from build123d import *

# Parameters (mm, degrees)
ESQUISSE1_W             = 30
ESQUISSE1_H             = 11
BOSS_EXTRU_1_DEPTH      = 16.2
BOSS_EXTRU_2_DEPTH      = 9.1
ESQUISSE3_W             = 33.4
ESQUISSE3_H             = 14
BOSS_EXTRU_3_DEPTH      = 2
CONG_1_R                = 3.5
ENL_V_MAT_EXTRU_1_DEPTH = 0.5


with BuildPart() as part:
    # Esquisse1 → Boss.-Extru.1 (new body)
    with BuildSketch(Plane.XY):
        Rectangle(ESQUISSE1_W, ESQUISSE1_H)
    extrude(amount=BOSS_EXTRU_1_DEPTH)

    # Esquisse2 → Boss.-Extru.2 (add)
    with BuildSketch(Plane(origin=(0, 0, 0), x_dir=(-1, 0, 0), z_dir=(0, 0, -1))):
        Polygon((-9.520156546, -2.694554874), (-13.5, 2.189177928), (-12.879843454, 2.694554874), (-8.9, -2.189177928), align=None)
        Polygon((-0.320156546, -2.694554874), (-4.3, 2.189177928), (-3.679843454, 2.694554874), (0.3, -2.189177928), align=None)
    extrude(amount=BOSS_EXTRU_2_DEPTH)

    # Esquisse3 → Boss.-Extru.3 (add)
    with BuildSketch(Plane.XY.offset(16.2)):
        Rectangle(ESQUISSE3_W, ESQUISSE3_H)
    extrude(amount=BOSS_EXTRU_3_DEPTH)

    # Congé1
    cong_1_edges = [part.edges().sort_by_distance(p)[0] for p in [
        (16.7, -7, 17.2),
        (16.7, 7, 17.2),
        (-16.7, 7, 17.2),
        (-16.7, -7, 17.2),
    ]]
    fillet(cong_1_edges, radius=CONG_1_R)

    # Esquisse5 → Enlèv. mat.-Extru.1 (cut)
    # profile 1 of 2: a face of its own
    with BuildSketch(Plane.XY.offset(18.2)):
        with BuildLine():
            add(Edge.make_bspline(
                [(-8.672344116, -3.115384615), (-8.816594542, -3.11454114), (-9.096803073, -3.112902677), (-9.505106438, -3.094675309), (-9.888147182, -3.064395858), (-10.245943635, -3.022899755), (-10.578588179, -2.972402097), (-10.885191819, -2.904990826), (-11.167173735, -2.828329399), (-11.425453052, -2.739480033), (-11.663510816, -2.639226475), (-11.885744181, -2.530107135), (-12.0918336, -2.40780713), (-12.285008724, -2.279261226), (-12.462319222, -2.139465144), (-12.62580805, -1.99141638), (-12.774096473, -1.832153938), (-12.907286041, -1.663222517), (-13.024073857, -1.485767046), (-13.127578093, -1.304636715), (-13.212833981, -1.116595132), (-13.282575645, -0.924117757), (-13.339507374, -0.72679892), (-13.378613639, -0.524688996), (-13.403175484, -0.317319479), (-13.405526699, -0.177353753), (-13.406719116, -0.106370192)],
                knots=[0, 0, 0, 0, 1.646148282, 3.197666765, 4.66315463, 6.030252048, 7.307778049, 8.501004361, 9.610818041, 10.641065266, 11.615491391, 12.557119604, 13.464013759, 14.348536654, 15.203310953, 16.038349431, 16.863300206, 17.683791446, 18.490318933, 19.285717724, 20.06220424, 20.843281102, 21.620494212, 22.403315558, 23.190242141, 24, 24, 24, 24], degree=3))
            add(Edge.make_bspline(
                [(-13.406719116, -0.106370192), (-13.405725902, -0.034758535), (-13.403749756, 0.107723458), (-13.375934308, 0.317616697), (-13.340032104, 0.523853953), (-13.28245088, 0.7233062), (-13.213547479, 0.919744698), (-13.122630536, 1.108284414), (-13.0237513, 1.295581798), (-12.90312695, 1.47312818), (-12.769817193, 1.646228322), (-12.618476538, 1.808491632), (-12.453293353, 1.964065993), (-12.270583572, 2.107075425), (-12.073148677, 2.243649111), (-11.859333594, 2.368602577), (-11.629612167, 2.484534626), (-11.385049352, 2.593624475), (-11.119112495, 2.689020666), (-10.833460316, 2.773835506), (-10.525506096, 2.843355619), (-10.196965336, 2.90084753), (-9.846210449, 2.945472196), (-9.473952104, 2.977949275), (-9.079957413, 2.995110587), (-8.810580002, 2.99834183), (-8.672344116, 3)],
                knots=[0, 0, 0, 0, 0.810910589, 1.61342667, 2.396193133, 3.181089899, 3.963115317, 4.752255436, 5.550715454, 6.36105385, 7.181178335, 8.024612154, 8.872680183, 9.750181803, 10.651284446, 11.591556747, 12.554036451, 13.566402641, 14.62422919, 15.753422176, 16.94128843, 18.199818041, 19.531985927, 20.947085226, 22.433341622, 24, 24, 24, 24], degree=3))
            add(Edge.make_bspline(
                [(-8.672344116, 3), (-8.534712415, 2.998305349), (-8.265942373, 2.994995999), (-7.873701987, 2.978317337), (-7.503450196, 2.944678932), (-7.154792256, 2.903215364), (-6.827566515, 2.845080871), (-6.521986194, 2.775033615), (-6.2369694, 2.695225184), (-5.974558239, 2.598364918), (-5.730419815, 2.491814224), (-5.502387515, 2.376006578), (-5.288628898, 2.251758245), (-5.090673237, 2.117232847), (-4.908696823, 1.971871056), (-4.74294709, 1.816405738), (-4.590643844, 1.652725679), (-4.455865409, 1.478616394), (-4.334322685, 1.299416276), (-4.231855178, 1.112099864), (-4.143073095, 0.921461088), (-4.070485552, 0.725596603), (-4.014193065, 0.524808811), (-3.975495046, 0.318430198), (-3.948293311, 0.107693838), (-3.9462218, -0.034768443), (-3.945180655, -0.106370192)],
                knots=[0, 0, 0, 0, 1.561645053, 3.049612875, 4.452756685, 5.778837748, 7.032101753, 8.221335837, 9.334924186, 10.387562255, 11.392109817, 12.355697819, 13.287721948, 14.19548756, 15.068665045, 15.927346723, 16.771751757, 17.602390507, 18.423119567, 19.225778204, 20.022010933, 20.807278863, 21.593079439, 22.384715467, 23.188155646, 24, 24, 24, 24], degree=3))
            add(Edge.make_bspline(
                [(-3.945180655, -0.106370192), (-3.946379855, -0.1773522), (-3.948744442, -0.317314863), (-3.973208323, -0.524706815), (-4.012539618, -0.726004524), (-4.067610881, -0.922201329), (-4.13502048, -1.114303766), (-4.22284416, -1.299694332), (-4.323989205, -1.480433653), (-4.439176304, -1.65604218), (-4.571150652, -1.823209934), (-4.717099564, -1.982916346), (-4.880765666, -2.131001619), (-5.059572209, -2.269585542), (-5.253034743, -2.399490408), (-5.461283099, -2.520733579), (-5.684672864, -2.632141235), (-5.924612019, -2.734107607), (-6.184724486, -2.824512173), (-6.467425199, -2.904059364), (-6.775585556, -2.967591262), (-7.107640965, -3.021444367), (-7.464266137, -3.064597565), (-7.845590095, -3.094662735), (-8.250888737, -3.11288884), (-8.529295376, -3.114537509), (-8.672344116, -3.115384615)],
                knots=[0, 0, 0, 0, 0.810927267, 1.598990287, 2.382942141, 3.152806972, 3.926217614, 4.706701772, 5.493896336, 6.292070767, 7.104102563, 7.925577746, 8.761822141, 9.623241997, 10.509042271, 11.423174113, 12.375371989, 13.360203808, 14.400680605, 15.520553799, 16.714061498, 17.994519714, 19.364400916, 20.818312473, 22.365209998, 24, 24, 24, 24], degree=3))
        make_face()
        with BuildLine():
            add(Edge.make_bspline(
                [(-8.675949886, -2.307692308), (-8.555739426, -2.307378423), (-8.32243453, -2.306769235), (-7.984001554, -2.291315187), (-7.667814755, -2.269804728), (-7.373997537, -2.242743333), (-7.103576783, -2.202215046), (-6.855428255, -2.156233227), (-6.630011273, -2.10108084), (-6.425355958, -2.035503901), (-6.238564308, -1.960805385), (-6.064657667, -1.879390931), (-5.901574914, -1.791153635), (-5.749711712, -1.694284826), (-5.610924423, -1.58686934), (-5.481695105, -1.47388697), (-5.366518241, -1.350247925), (-5.228358565, -1.179245905), (-5.085597394, -0.953479952), (-4.961278178, -0.669028437), (-4.883152037, -0.376737863), (-4.873216642, -0.17834897), (-4.868257578, -0.079326923)],
                knots=[0, 0, 0, 0, 1.459098681, 2.831824031, 4.11146945, 5.306290378, 6.412266529, 7.42953815, 8.369053297, 9.227277979, 10.03601793, 10.809473603, 11.557037441, 12.285528272, 12.993193355, 13.685654407, 14.36688038, 15.041354379, 16.352855396, 17.594313975, 18.799247529, 20, 20, 20, 20], degree=3))
            add(Edge.make_bspline(
                [(-4.868257578, -0.079326923), (-4.872599831, 0.020268324), (-4.881268934, 0.219105532), (-4.956929449, 0.511127608), (-5.079929419, 0.792278573), (-5.220453969, 1.014159934), (-5.355136893, 1.182494904), (-5.469834642, 1.303148633), (-5.598299711, 1.413876824), (-5.736895921, 1.518900078), (-5.88828286, 1.615223199), (-6.051729325, 1.702814186), (-6.227690112, 1.782742777), (-6.350526578, 1.828280326), (-6.413329693, 1.8515625)],
                knots=[0, 0, 0, 0, 1.353621445, 2.702441307, 4.075953605, 5.516772412, 6.261413105, 7.007624062, 7.778524365, 8.566925914, 9.372323995, 10.217594641, 11.088702136, 12, 12, 12, 12], degree=3))
            add(Edge.make_bspline(
                [(-6.413329693, 1.8515625), (-6.493634738, 1.878695617), (-6.656688417, 1.933787481), (-6.909623522, 2.004789187), (-7.175002058, 2.060705927), (-7.451238073, 2.111011725), (-7.740368732, 2.145348154), (-8.041499434, 2.172985389), (-8.354857222, 2.189264298), (-8.567758628, 2.191282229), (-8.675949886, 2.192307692)],
                knots=[0, 0, 0, 0, 0.884706709, 1.796334032, 2.740027952, 3.714592787, 4.726048262, 5.777819803, 6.87074269, 8, 8, 8, 8], degree=3))
            add(Edge.make_bspline(
                [(-8.675949886, 2.192307692), (-8.784123643, 2.19089292), (-8.995734639, 2.188125323), (-9.305638532, 2.177546497), (-9.599984203, 2.150228735), (-9.880039702, 2.119888142), (-10.144254773, 2.075152436), (-10.394841251, 2.026918055), (-10.628694816, 1.962115009), (-10.849476345, 1.892892484), (-11.054678905, 1.813666605), (-11.245254183, 1.726451773), (-11.422139784, 1.633320403), (-11.584789178, 1.53211866), (-11.734145807, 1.424256181), (-11.866772982, 1.305865626), (-11.989122286, 1.184465672), (-12.12628489, 1.011809345), (-12.267242107, 0.787609853), (-12.393430821, 0.506705562), (-12.468112707, 0.21598173), (-12.47846943, 0.019038319), (-12.483642193, -0.079326923)],
                knots=[0, 0, 0, 0, 1.313483664, 2.569454835, 3.763100662, 4.901599063, 5.988328865, 7.015709358, 7.99797933, 8.932480776, 9.824041341, 10.666387587, 11.475829342, 12.24921787, 12.990555181, 13.709176526, 14.405678811, 15.080244297, 16.38186033, 17.610124501, 18.806354173, 20, 20, 20, 20], degree=3))
            add(Edge.make_bspline(
                [(-12.483642193, -0.079326923), (-12.478456561, -0.178883567), (-12.468075849, -0.378178222), (-12.393776202, -0.672006713), (-12.267611311, -0.954808682), (-12.12655646, -1.179747502), (-11.989648182, -1.350306344), (-11.873123474, -1.471338898), (-11.74698074, -1.585888179), (-11.606962249, -1.690522154), (-11.455634138, -1.786816559), (-11.29466033, -1.87846391), (-11.120428745, -1.958789639), (-10.933783565, -2.033727971), (-10.729116994, -2.099414291), (-10.502884375, -2.1539365), (-10.254143251, -2.203572524), (-9.981746648, -2.239318551), (-9.687866721, -2.270795303), (-9.370871329, -2.291079041), (-9.031276204, -2.30684003), (-8.796764226, -2.307402525), (-8.675949886, -2.307692308)],
                knots=[0, 0, 0, 0, 1.207546505, 2.417292871, 3.651582144, 4.952510111, 5.626719005, 6.30238548, 6.989136872, 7.692112372, 8.420316868, 9.164734959, 9.937886623, 10.746308695, 11.604196049, 12.543341915, 13.568754172, 14.680483261, 15.875568977, 17.154711427, 18.534182925, 20, 20, 20, 20], degree=3))
        make_face(mode=Mode.SUBTRACT)
    # profile 2 of 2: a face of its own
    with BuildSketch(Plane.XY.offset(18.2)):
        Polygon((2.670203961, -1.202524038), (2.670203961, 0.461538462), (11.670203961, 0.461538462), (11.670203961, -0.346153846), (3.593280884, -0.346153846), (3.593280884, -1.730769231), align=None)
    extrude(amount=-ENL_V_MAT_EXTRU_1_DEPTH, mode=Mode.SUBTRACT)


solid = part.part
Check sheet for the modelled part. Datum: model origin and axes. Units: mm. A direction names the side the tool comes from. Give positions to 0.01 mm unless a question says otherwise; leave off trailing zeros. Order: outer loops, then holes, each group sorted by start corner. A loop starts at its lowest first (then second) coordinate and runs counter-clockwise, first axis right, second up. Notation, with made-up numbers: M 16,-15.5 L 33,-15.5 A7 ccw 33,-3.5 Z; hole C 47.5,86 d3. An arc over 180 degrees is marked long. Answer as CSV lines item,"result". Start each with the question number.
Item 1: Mould release check, pull along X, two halves, no side actions. Record for faces 4 (the face through (2, 0, -9.1)), 5 (the face through (2.28, -0.29, -4.49)), 6 (the face through (-16.7, 0, 17)): +X half, -X half, draft (parallel to the pull), parting line (faces both ways), or undercut.
Item 2: Cross-section at B-B on x = 5.5. Enter the section's corners in (y, z), plus the area to 3 significant figures.
Item 3: Gauge pin test, flat ends, axial feed: P1, Ø4, axis at y = -1.5, z = 1.5, coming from the +X side; P2, Ø1.5, axis at x = 0, z = 1, coming from the -Y side; P3, Ø5, axis at x = -9, z = 7.5, coming from the +Y side. Record the tip position at first contact, or that the pin passes through.
Item 4: Cross-section at D-D on z = 13.25. Enter the section's corners in (x, y).
Item 5: Tool access check on faces 1 (the face through (-8.3, -2.5, 17.7)), 2 (the face through (-15, 0, 8)), 3 (the face through (1.72, 0.29, -4.49)). Record the directions out of +Z, -Z, +X, -X, +Y, -Y that give a thin tool (end or side, any length) a straight path to the whole face; none if there is none.
Item 6: Thickness scan on line 1 (Z direction, x = -7, y = -1.75); line 2 (Y direction, x = 5, z = 8.75); line 3 (Z direction, x = -5, y = 6). Record the ranges inside material, lowest first. Write a range as [from, to].
Item 7: Cross-section at C-C on y = 5. Enter the section's corners in (x, z).
Item 8: Cross-section at A-A on z = -5.75. Enter the section's corners in (x, y), plus the area to 3 significant figures.
Established:
1,face 4,"draft"
1,face 5,"undercut"
1,face 6,"-X half"
2,outline,"M -7,16.2 L -5.5,16.2 L -5.5,0 L 5.5,0 L 5.5,16.2 L 7,16.2 L 7,18.2 L 0.46,18.2 L 0.46,17.7 L -0.35,17.7 L -0.35,18.2 L -7,18.2 Z"
2,area,"206 mm^2"
3,P1,"stops at x = 15"
3,P2,"stops at y = -5.5"
3,P3,"stops at y = 5.5"
4,outline,"M -15,-5.5 L 15,-5.5 L 15,5.5 L -15,5.5 Z"
5,face 1,"+Z"
5,face 2,"-Z, -X, +Y, -Y"
5,face 3,"-Z, -X, +Y"
6,line 1,"z = [0, 18.2]"
6,line 2,"y = [-5.5, 5.5]"
6,line 3,"z = [16.2, 18.2]"
7,outline,"M -16.36,16.2 L -15,16.2 L -15,0 L 15,0 L 15,16.2 L 16.36,16.2 L 16.36,18.2 L -16.36,18.2 Z"
8,outline,"M -0.3,-2.19 L 0.32,-2.69 L 4.3,2.19 L 3.68,2.69 Z; M 8.9,-2.19 L 9.52,-2.69 L 13.5,2.19 L 12.88,2.69 Z"
8,area,"10.1 mm^2"
